Verification items for this drawing (mm, ordinates from the low corner). A direction names the side the tool comes from. Coordinates: 2 decimals unless noted, no trailing zeros. Order: outer loops, then holes, each group sorted by start corner. A loop starts at its lowest first (then second) coordinate and runs counter-clockwise, first axis right, second up. Notation, with made-up numbers: M -14,-20 L 24,-20 A32 cw 24,12 Z; hole C -7.5,87.25 d5. An arc over 180 degrees is marked long. Answer as a JSON object with one key per item and string values. Group by question number.
(1) Access from +Z, -Z, +X, -X, +Y, -Y to the whole of each face (thin tool, end or side, straight path). Record for the marked faces 4 and 5.
(2) Gauge pin test, flat ends, axial feed: pin 1 Ø5.5 at (y, z) = (9.13, 21.92) entering from +X (3 decimals); pin 2 Ø1 at (y, z) = (11.5, 13) entering from +X; pin 3 Ø2 at (x, z) = (6.5, 6.5) entering from +Y; pin 4 Ø6 at (x, z) = (11, 23) entering from -Y. Record the tip position at first contact, or that the pin passes through.
(3) Mould release check, pull along Y, two halves, no side actions. Record for the marked faces 1, 2 and 3: released by +Y, released by -Y, zero draft, split by the parting line, or undercut.
(4) Cross-section at C-C (z = 37). Enter the section's corners in (x, y) (1 decimal), plus the area to 3 significant figures.
(5) Material ranges on line 1 (Z direction, x = 16.25, y = 7); line 2 (X direction, y = 9.5, z = 9.5) (1 decimal); line 3 (Z direction, x = 14.5, y = 8.75), recorded low to high.
(6) Cross-section at B-B (x = 11.5). Enter the section's corners in (y, z).
(7) Cross-section at D-D (y = 11.5). Enter the section's corners in (x, z).
(8) Cross-section at A-A (y = 8.5). Enter the section's corners in (x, z).
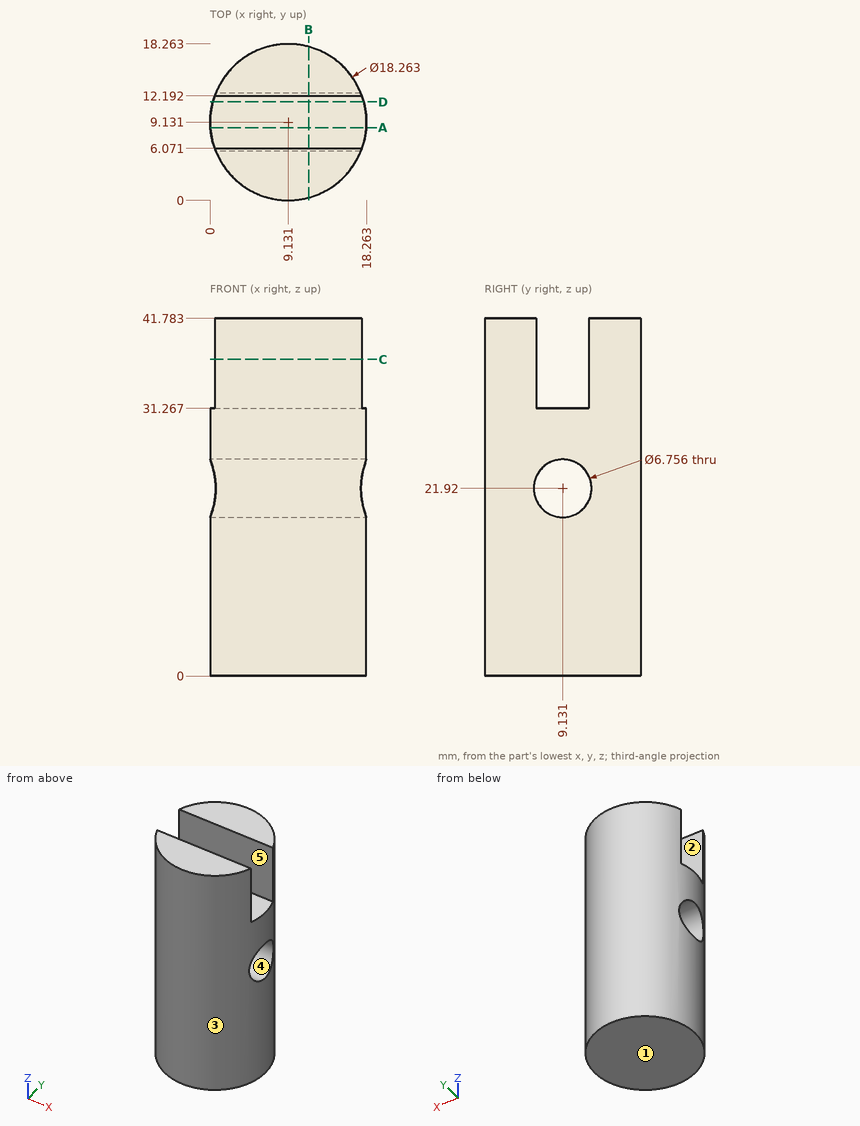
Taken from the geometry:
{
 "1": {"face 4": "+X, -X", "face 5": "+Z, +X, -X"},
 "2": {"pin 1": "passes through", "pin 2": "stops at x = 18.07", "pin 3": "stops at y = 18.12", "pin 4": "stops at y = 0"},
 "3": {"face 1": "zero draft", "face 2": "undercut", "face 3": "split by the parting line"},
 "4": {"outline": "M 0.5,6.1 A9.1 ccw 17.7,6.1 Z; M 0.5,12.2 L 17.7,12.2 A9.1 ccw Z", "area": "152 mm²"},
 "5": {"line 1": "z = 0 to 19.3, 24.54 to 31.27", "line 2": "x = 0 to 18.3", "line 3": "z = 0 to 18.56, 25.28 to 31.27"},
 "6": {"outline": "M 0.31,0 L 17.95,0 L 17.95,41.78 L 12.19,41.78 L 12.19,31.27 L 6.07,31.27 L 6.07,41.78 L 0.31,41.78 Z; hole C 9.13,21.92 d6.76"},
 "7": {"outline": "M 0.31,0 L 17.95,0 L 17.95,19.51 L 0.31,19.51 Z; M 0.31,24.33 L 17.95,24.33 L 17.95,31.27 L 0.31,31.27 Z"},
 "8": {"outline": "M 0.02,0 L 18.24,0 L 18.24,18.6 L 0.02,18.6 Z; M 0.02,25.24 L 18.24,25.24 L 18.24,31.27 L 0.02,31.27 Z"}
}
